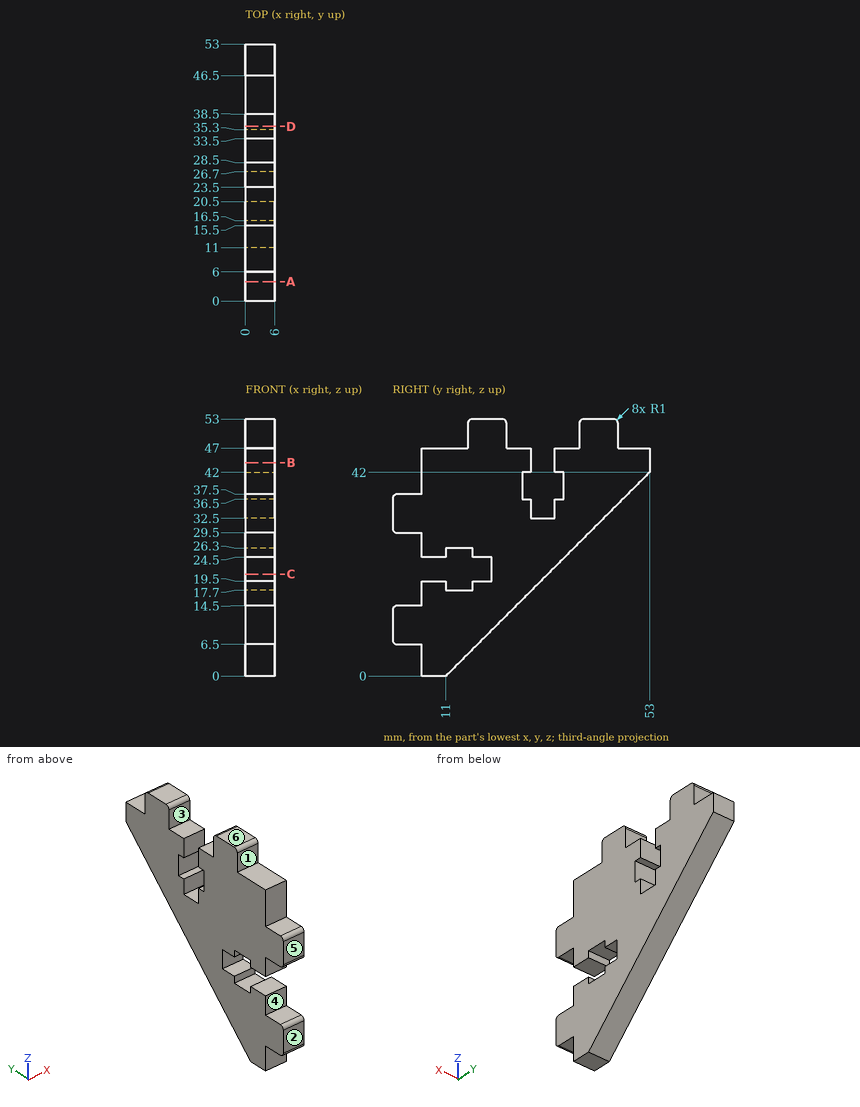
Input: dimensioned drawing with shaded views. Units: mm. Origin: part minimum x, y, z. A direction names the side the tool comes from. Round coordinates to 2 decimals unless told otherwise and drop trailing zeros. Loops run counter-clockwise (first coordinate to the right, second up) from the corner with the lowest first, then second, coordinate; pieces in that order, holes last. Notation, with made-up numbers: (81, -18) -> (124, -18) arc R31 ccw to (124, 13) -> close; hole circle Ø3 at (-19.75, -9). An arc over 180 degrees is marked (long way). Answer as a JSON object with one key per item and string values. Group by question number.
1) Reachability of the marked faces 1, 2 and 3 from +Z, -Z, +X, -X, +Y, -Y: full face, straight path, thin tool, end or side. Return the list, or none.
2) Pin query (flat end, axial travel): pin 1 (1.4 mm diameter, centred on x = 4, z = 25.5, fed in from +Y); pin 2 (2.5 mm diameter, centred on x = 4, z = 49.5, fed in from +Y); pin 3 (0.5 mm diameter, centred on x = 2.5, y = 27.5, fed in from -Z); pin 4 (12 mm diameter, centred on y = 43.5, z = 16, fed in from -X). Return the tip coordinate at first contact, or that it passes through.
3) Ray query, L1, parallel to Y at x = 4.8, z = 44; L2, parallel to Z at x = 4.45, y = 34.5; L3, parallel to Z at x = 1.6, y = 18.5. Return the intervals inside material, ascending.
4) Section query D-D on y = 36. Output: boundary loops of the cut face in (x, z), plus the area to 3 significant figures.
5) Section query A-A on y = 4. Output: boundary loops of the cut face in (x, z), plus the area to 3 significant figures.
6) Section query B-B on z = 44. Output: boundary loops of the cut face in (x, y), plus the area to 3 significant figures.
7) Section query C-C on z = 21. Output: boundary loops of the cut face in (x, y).
8) Draft query along Z for the marked faces 4, 5 and 6. Return one class per face: +Z half, -Z half, draft (parallel to the pull), parting line (faces both ways), or undercut.
Reply:
{
 "1": {"face 1": "+Z, +X, -X, -Y", "face 2": "+Z, -Z, +X, -X, -Y", "face 3": "+Z, +X, -X"},
 "2": {"pin 1": "stops at y = 37.2", "pin 2": "stops at y = 46.5", "pin 3": "stops at z = 16.25", "pin 4": "passes through"},
 "3": {"L1": "y = 6 to 28.5, 33.5 to 53", "L2": "z = 23.5 to 36.5, 42 to 47", "L3": "z = 7.5 to 19.5, 24.5 to 53"},
 "4": {"outline": "(0, 25) -> (6, 25) -> (6, 47) -> (0, 47) -> close", "area": "132 mm2"},
 "5": {"outline": "(0, 6.5) -> (6, 6.5) -> (6, 14.5) -> (0, 14.5) -> close; (0, 29.5) -> (6, 29.5) -> (6, 37.5) -> (0, 37.5) -> close", "area": "96.0 mm2"},
 "6": {"outline": "(0, 6) -> (6, 6) -> (6, 28.5) -> (0, 28.5) -> close; (0, 33.5) -> (6, 33.5) -> (6, 53) -> (0, 53) -> close", "area": "252 mm2"},
 "7": {"outline": "(0, 20.5) -> (6, 20.5) -> (6, 32) -> (0, 32) -> close"},
 "8": {"face 4": "undercut", "face 5": "draft", "face 6": "+Z half"}
}
